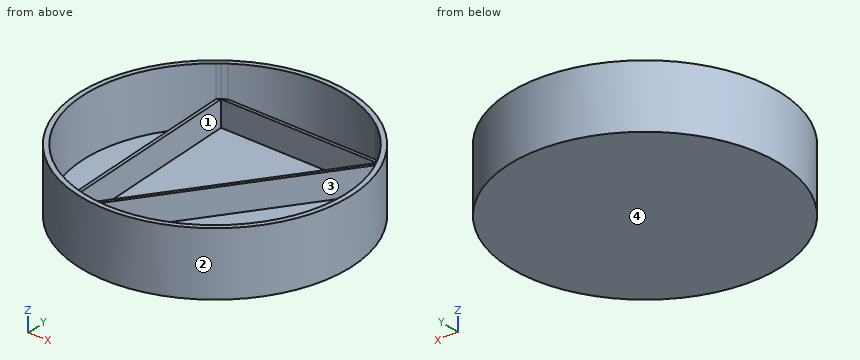
```python
from build123d import *

# Parameters (mm, degrees)
F0_R     = 21.007285
F1_DEPTH = 10
F2_DEPTH = 5
F3_DEPTH = 1


with BuildPart() as f1:
    # F0 (on Top) → F1 (new body)
    with BuildSketch(Plane.XY):
        with Locations((-22.267804, 31.613778)):
            Circle(F0_R)
        with BuildLine():
            ThreePointArc((-9.054285, 46.93661), (-3.872977, 40.040914), (-2.034508, 31.613778))
            ThreePointArc((-2.034508, 31.613778), (-12.277525, 14.018876), (-32.635611, 14.238658))
            ThreePointArc((-32.635611, 14.238658), (-32.851833, 14.369517), (-33.066404, 14.503066))
            ThreePointArc((-33.066404, 14.503066), (-33.325959, 14.669652), (-33.582945, 14.840174))
            ThreePointArc((-33.582945, 14.840174), (-42.48798, 30.885292), (-34.760672, 47.529634))
            ThreePointArc((-34.760672, 47.529634), (-34.516623, 47.718208), (-34.269729, 47.90304))
            ThreePointArc((-34.269729, 47.90304), (-33.927332, 48.149849), (-33.579861, 48.389463))
            ThreePointArc((-33.579861, 48.389463), (-21.7455, 51.840331), (-10.105014, 47.78328))
            ThreePointArc((-10.105014, 47.78328), (-9.770373, 47.526052), (-9.441171, 47.2619))
            ThreePointArc((-9.441171, 47.2619), (-9.246712, 47.100463), (-9.054285, 46.93661))
        make_face(mode=Mode.SUBTRACT)
    extrude(amount=F1_DEPTH)

    # F0 (on Top) → F2 (join)
    with BuildSketch(Plane.XY):
        with BuildLine():
            Line((-34.269729, 47.90304), (-9.441171, 47.2619))
            ThreePointArc((-9.441171, 47.2619), (-9.770373, 47.526052), (-10.105014, 47.78328))
            Line((-10.105014, 47.78328), (-33.579861, 48.389463))
            ThreePointArc((-33.579861, 48.389463), (-33.927332, 48.149849), (-34.269729, 47.90304))
        make_face()
        with BuildLine():
            Line((-32.635611, 14.238658), (-9.054285, 46.93661))
            ThreePointArc((-9.054285, 46.93661), (-9.246712, 47.100463), (-9.441171, 47.2619))
            Line((-9.441171, 47.2619), (-33.066404, 14.503066))
            ThreePointArc((-33.066404, 14.503066), (-32.851833, 14.369517), (-32.635611, 14.238658))
        make_face()
        with BuildLine():
            ThreePointArc((-33.582945, 14.840174), (-33.325959, 14.669652), (-33.066404, 14.503066))
            Line((-33.066404, 14.503066), (-34.269729, 47.90304))
            ThreePointArc((-34.269729, 47.90304), (-34.516623, 47.718208), (-34.760672, 47.529634))
            Line((-34.760672, 47.529634), (-33.582945, 14.840174))
        make_face()
    extrude(amount=F2_DEPTH)

    # F0 (on Top) → F3 (join)
    with BuildSketch(Plane.XY):
        Polygon((-33.066404, 14.503066), (-9.441171, 47.2619), (-34.269729, 47.90304), align=None)
        with BuildLine():
            Line((-33.579861, 48.389463), (-10.105014, 47.78328))
            ThreePointArc((-10.105014, 47.78328), (-21.7455, 51.840331), (-33.579861, 48.389463))
        make_face()
        with BuildLine():
            ThreePointArc((-32.635611, 14.238658), (-12.277525, 14.018876), (-2.034508, 31.613778))
            ThreePointArc((-2.034508, 31.613778), (-3.872977, 40.040914), (-9.054285, 46.93661))
            Line((-9.054285, 46.93661), (-32.635611, 14.238658))
        make_face()
        with BuildLine():
            ThreePointArc((-34.760672, 47.529634), (-42.48798, 30.885292), (-33.582945, 14.840174))
            Line((-33.582945, 14.840174), (-34.760672, 47.529634))
        make_face()
    extrude(amount=F3_DEPTH)


solid = f1.part
```
Part model, mm, in its own coordinate system. Face numbers are marked on the shaded views. Round coordinates to 2 decimals unless told otherwise and drop trailing zeros. Loops run counter-clockwise (first coordinate to the right, second up) from the corner with the lowest first, then second, coordinate; pieces in that order, holes last.
1. Slice it at A-A (z = 5.75). Give the cut face in (x, y).
Solutions:
outline: circle Ø42.01 at (-22.27, 31.61); hole (-34.76, 47.53) arc R20.23 ccw to (-33.58, 14.84) arc R20.24 ccw to (-33.07, 14.5) arc R20.24 ccw to (-32.64, 14.24) arc R20.23 ccw to (-2.03, 31.61) arc R20.23 ccw to (-9.05, 46.94) arc R20.23 ccw to (-9.44, 47.26) arc R20.23 ccw to (-10.11, 47.78) arc R20.23 ccw to (-33.58, 48.39) arc R20.23 ccw to (-34.27, 47.9) arc R20.24 ccw to start
2. Two-plate mould, pull along Y, no slides. Class the marked faces 1, 2, 3 and 4: pulls with the +Y half, pulls with the -Y half, needs draft (parallel to the pull), parting line crosses it, or undercut.
Solutions:
face 1: undercut
face 2: parting line crosses it
face 3: undercut
face 4: needs draft
3. Slice it at C-C (y = 18). Give the cut face in (x, z).
Solutions:
outline: (-38.27, 0) - (-6.27, 0) - (-6.27, 10) - (-7.3, 10) - (-7.3, 1) - (-29.92, 1) - (-29.92, 5) - (-30.54, 5) - (-30.54, 1) - (-33.19, 1) - (-33.19, 5) - (-33.7, 5) - (-33.7, 1) - (-37.24, 1) - (-37.24, 10) - (-38.27, 10) - close
4. Slice it at D-D (x = -37.5). Give the cut face in (y, z).
Solutions:
outline: (17.15, 0) - (46.08, 0) - (46.08, 10) - (44.93, 10) - (44.93, 1) - (18.3, 1) - (18.3, 10) - (17.15, 10) - close
5. Slice it at B-B (z = 2). Give the cut face in (x, y), and give its area (3 significant figures).
Solutions:
outline: circle Ø42.01 at (-22.27, 31.61); hole (-34.76, 47.53) arc R20.23 ccw to (-33.58, 14.84) - close; hole (-34.27, 47.9) - (-33.07, 14.5) - (-9.44, 47.26) - close; hole (-33.58, 48.39) - (-10.11, 47.78) arc R20.23 ccw to start; hole (-32.64, 14.24) arc R20.23 ccw to (-2.03, 31.61) arc R20.23 ccw to (-9.05, 46.94) - close
area: 149 mm2
6. Drill centre lines: line 1 along Y through (x, z) = (-18.5, 1.25); line 2 along Y through (x, z) = (-27.5, 3.5); line 3 along Y through (x, z) = (-10, 3.25). Where is each one in solid material? Low to high.
Solutions:
line 1: y = 10.95 to 11.73, 33.84 to 34.7, 47.5 to 48, 51.49 to 52.28
line 2: y = 11.27 to 12.07, 21.36 to 22.22, 47.73 to 48.23, 51.16 to 51.96
line 3: y = 14.56 to 15.52, 45.63 to 46.49, 47.28 to 48.67
7. Flat gauge pins, fed straight in: pin 1 (1.5 mm diameter, centred on x = -38.5, y = 32, fed in from +Z); pin 2 (19 mm diameter, centred on x = -21.5, y = 27, fed in from +Z); pin 3 (2 mm diameter, centred on x = -36, z = 1.5, fed in from -Y). Where does each tip first touch, or does it go through?
Solutions:
pin 1: stops at z = 1
pin 2: stops at z = 5
pin 3: stops at y = 14.9
